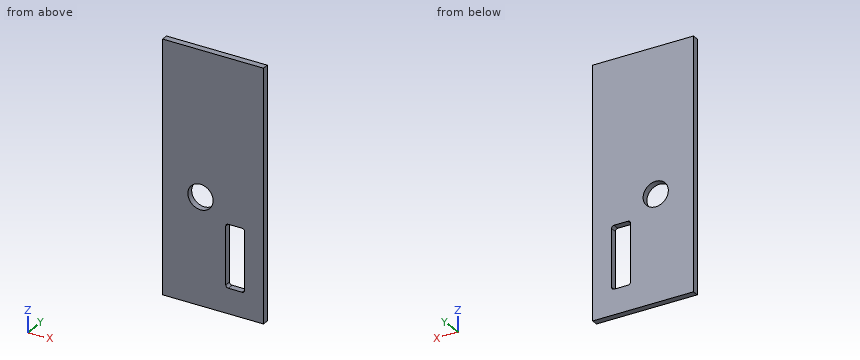
from build123d import *

# Parameters (mm, degrees)
SKETCH1_W           = 101.6
SKETCH1_H           = 254
SKETCH1_R           = 12.7
BOSS_EXTRUDE1_DEPTH = 6.35


with BuildPart() as part:
    # Sketch1 → Boss-Extrude1 (new body)
    with BuildSketch(Plane(origin=(0, 0, 0), x_dir=(1, 0, 0), z_dir=(0, 1, 0))):
        Rectangle(SKETCH1_W, SKETCH1_H)
        with Locations((-12.7, 19.05)):
            Circle(SKETCH1_R, mode=Mode.SUBTRACT)
        with BuildLine():
            Line((29.21, 101.6), (15.24, 101.6))
            ThreePointArc((15.24, 101.6), (13.443948776, 100.856051224), (12.7, 99.06))
            Line((12.7, 99.06), (12.7, 40.64))
            ThreePointArc((12.7, 40.64), (13.443948776, 38.843948776), (15.24, 38.1))
            Line((15.24, 38.1), (29.21, 38.1))
            ThreePointArc((29.21, 38.1), (31.006051224, 38.843948776), (31.75, 40.64))
            Line((31.75, 40.64), (31.75, 99.06))
            ThreePointArc((31.75, 99.06), (31.006051224, 100.856051224), (29.21, 101.6))
        make_face(mode=Mode.SUBTRACT)
    extrude(amount=BOSS_EXTRUDE1_DEPTH)


solid = part.part
Model file for the job. Use its own axes, mm. Give positions to 0.01 mm unless a question says otherwise; leave off trailing zeros. Loops run counter-clockwise (first coordinate to the right, second up) from the corner with the lowest first, then second, coordinate; pieces in that order, holes last.
Item 1: Slice it at C-C (y = 4). Write the cut outline in (x, z), plus the area to 3 significant figures.
Check values:
outline: (-50.8, -127) - (50.8, -127) - (50.8, 127) - (-50.8, 127) - close; hole circle Ø25.4 at (-12.7, -19.05); hole (12.7, -99.06) arc R2.54 ccw to (15.24, -101.6) - (29.21, -101.6) arc R2.54 ccw to (31.75, -99.06) - (31.75, -40.64) arc R2.54 ccw to (29.21, -38.1) - (15.24, -38.1) arc R2.54 ccw to (12.7, -40.64) - close
area: 24,100 mm2
Item 2: Slice it at B-B (z = -19.05). Write the cut outline in (x, y).
Check values:
outline: (-50.8, 0) - (-25.4, 0) - (-25.4, 6.35) - (-50.8, 6.35) - close; (0, 0) - (50.8, 0) - (50.8, 6.35) - (0, 6.35) - close
Item 3: Drill centre lines: line 1 along X through (y, z) = (4, -19.05); line 2 along Z through (x, y) = (-12.7, 2.5); line 3 along X through (y, z) = (3.75, -99.5). Where is each one in solid material? Low to high.
Check values:
line 1: x = -50.8 to -25.4, 0 to 50.8
line 2: z = -127 to -31.75, -6.35 to 127
line 3: x = -50.8 to 12.74, 31.71 to 50.8
Item 4: Slice it at A-A (x = -12.7). Write the cut outline in (y, z), plus the area to 3 significant figures.
Check values:
outline: (0, -127) - (6.35, -127) - (6.35, -31.75) - (0, -31.75) - close; (0, -6.35) - (6.35, -6.35) - (6.35, 127) - (0, 127) - close
area: 1,450 mm2
